Design review of the part built by this model. Coordinates are the model's own, in mm. A direction names the side the tool comes from. Give positions to 0.01 mm unless a question says otherwise; leave off trailing zeros. Order: outer loops, then holes, each group sorted by start corner. A loop starts at its lowest first (then second) coordinate and runs counter-clockwise, first axis right, second up. Notation, with made-up numbers: M -39.5,50 L -28.5,50 A28 ccw -28.5,78 Z; hole C 57,-39.75 d3. An arc over 180 degrees is marked long. Answer as a JSON object with one key per item and string values.
from build123d import *

# Parameters (mm, degrees)
SKETCH1_R           = 64
BOSS_EXTRUDE1_DEPTH = 6
SKETCH2_R           = 7.25
BOSS_EXTRUDE2_DEPTH = 20
SKETCH3_R           = 5
BOSS_EXTRUDE3_DEPTH = 15
SKETCH4_R           = 1.9
CUT_EXTRUDE1_DEPTH  = 10


with BuildPart() as part:
    # Sketch1 → Boss-Extrude1 (new body)
    with BuildSketch(Plane(origin=(0, 0, 0), x_dir=(1, 0, 0), z_dir=(0, 1, 0))):
        with Locations(Location((0, 0, 0), (0, 0, 270))):
            Circle(SKETCH1_R)
    extrude(amount=BOSS_EXTRUDE1_DEPTH)

    # Sketch2 → Boss-Extrude2 (add)
    with BuildSketch(Plane.XZ):
        with Locations(Location((0, 0, 0), (0, 0, 90))):
            Circle(SKETCH2_R)
    extrude(amount=BOSS_EXTRUDE2_DEPTH)

    # Sketch3 → Boss-Extrude3 (add)
    with BuildSketch(Plane.XZ.offset(20)):
        with Locations(Location((0, 0, 0), (0, 0, 270))):
            Circle(SKETCH3_R)
    extrude(amount=BOSS_EXTRUDE3_DEPTH)

    # Sketch4 → Cut-Extrude1 (cut, symmetric)
    with BuildSketch(Plane(origin=(0, 0, 0), x_dir=(0, 0, -1), z_dir=(1, 0, 0))):
        with Locations(Location((0, -31, 0), (0, 0, 180))):
            Circle(SKETCH4_R)
        with Locations(Location((0, -24, 0), (0, 0, 180))):
            Circle(SKETCH4_R)
    extrude(amount=CUT_EXTRUDE1_DEPTH, both=True, mode=Mode.SUBTRACT)


solid = part.part
(1) To check wall thickness, follow L1, parallel to Y at x = 1, z = 0; L2, parallel to Y at x = -6, z = 8; L3, parallel to Z at x = 1.7, y = -31. State the ranges of each line that lie inside material, in increasing order. Write a range as from..to.
Checked values:
{"L1": "y = -35..-32.9, -29.1..-25.9, -22.1..6", "L2": "y = 0..6", "L3": "z = -4.7..-1.9, 1.9..4.7"}
(2) We need section A-A (z = 0). Write out the cut boundary in (x, y).
Checked values:
{"outline": "M -64,0 L -7.25,0 L -7.25,-20 L -5,-20 L -5,-22.1 L 5,-22.1 L 5,-20 L 7.25,-20 L 7.25,0 L 64,0 L 64,6 L -64,6 Z; M -5,-35 L 5,-35 L 5,-32.9 L -5,-32.9 Z; M -5,-29.1 L 5,-29.1 L 5,-25.9 L -5,-25.9 Z"}
(3) Draft analysis for pull direction Y (two halves, no side actions). For faces 1 (the cylindrical face through (2.777, -9.86, 6.697)), 2 (the cylindrical face through (0.07, -25.884, -0.247)), 3 (the flat face through (5, -20, -2)), state which applies: +Y half, -Y half, draft (parallel to the pull), parting line (faces both ways), or undercut.
Checked values:
{"face 1": "draft", "face 2": "undercut", "face 3": "-Y half"}
(4) Insertion check: pin 1 (1 mm diameter, centred on x = -17.5, z = -42.5, fed in from -Y); pin 2 (4.5 mm diameter, centred on y = -31, z = 0, fed in from -X); pin 3 (2 mm diameter, centred on y = 0, z = 3.5, fed in from +X). Each pin has a flat end and moves straight along its axis. Give the tip position at first contact, or say it passes through.
Checked values:
{"pin 1": "stops at y = 0", "pin 2": "stops at x = -5", "pin 3": "stops at x = 63.95"}
(5) We need section D-D (y = -31). Write out the cut boundary in (x, z).
Checked values:
{"outline": "M -4.62,-1.9 A5 ccw 4.62,-1.9 Z; M -4.62,1.9 L 4.62,1.9 A5 ccw Z"}
(6) We need section C-C (x = -52.5). Write out the cut boundary in (y, z), plus the area to 3 significant figures.
Checked values:
{"outline": "M 0,-36.6 L 6,-36.6 L 6,36.6 L 0,36.6 Z", "area": "439 mm^2"}
(7) Tool access review of faces 4 (the cylindrical face through (-4.436, -27.395, -2.307)), 5 (the flat face through (1, 6, -1)): name each direction out of +Z, -Z, +X, -X, +Y, -Y from which nothing blocks a thin tool from reaching the whole face with its end or side.
Checked values:
{"face 4": "-Y", "face 5": "+Z, -Z, +X, -X, +Y"}
(8) We need section B-B (y = -1.5). Write out the cut boundary in (x, z), plus the area to 3 significant figures.
Checked values:
{"outline": "C 0,0 d14.5", "area": "165 mm^2"}
